Design review of the part built by this model. Coordinates are the model's own, in mm. A direction names the side the tool comes from. Coordinates: 2 decimals unless noted, no trailing zeros. Write each loop counter-clockwise with the first axis right and the second up, starting at its lowest first coordinate (ties: lowest second). Pieces come first, ordered by that corner, then holes. Notation, with made-up numbers: (-36, 79) - (-30, 79) arc R16 ccw to (-30, 89) - close; hole circle Ø1 at (22.25, -5.5). An arc over 180 degrees is marked (long way). One line per item, written item: value.
from build123d import *

# Parameters (mm, degrees)
SCHIZZO1_R                   = 1.5
ESTRUSIONE_ESTRUSIONE1_DEPTH = 4


with BuildPart() as part:
    # Schizzo1 → Estrusione-Estrusione1 (new body)
    with BuildSketch(Plane.XY):
        with BuildLine():
            Line((22.627416998, 28.387976608), (-22.627416998, 28.387976608))
            ThreePointArc((-22.627416998, 28.387976608), (-27.949480117, 24.831887722), (-26.700747761, 18.554086235))
            Line((-26.700747761, 18.554086235), (-4.073330763, -4.073330763))
            ThreePointArc((-4.073330763, -4.073330763), (0, -5.76055961), (4.073330763, -4.073330763))
            Line((4.073330763, -4.073330763), (26.700747761, 18.554086235))
            ThreePointArc((26.700747761, 18.554086235), (27.949480117, 24.831887722), (22.627416998, 28.387976608))
        make_face()
        Circle(SCHIZZO1_R, mode=Mode.SUBTRACT)
        with Locations((22.627416998, 22.627416998)):
            Circle(SCHIZZO1_R, mode=Mode.SUBTRACT)
        with Locations((-22.627416998, 22.627416998)):
            Circle(SCHIZZO1_R, mode=Mode.SUBTRACT)
        with BuildLine():
            Line((5.727922061, 17.627416998), (-5.727922061, 17.627416998))
            ThreePointArc((-5.727922061, 17.627416998), (-7.575681126, 16.392783863), (-7.142135624, 14.213203436))
            Line((-7.142135624, 14.213203436), (-1.414213562, 8.485281374))
            ThreePointArc((-1.414213562, 8.485281374), (0, 7.899494937), (1.414213562, 8.485281374))
            Line((1.414213562, 8.485281374), (7.142135624, 14.213203436))
            ThreePointArc((7.142135624, 14.213203436), (7.575681126, 16.392783863), (5.727922061, 17.627416998))
        make_face(mode=Mode.SUBTRACT)
    extrude(amount=ESTRUSIONE_ESTRUSIONE1_DEPTH)


solid = part.part
1. Consider section A-A, the plane z = 0.75. Write out the cut boundary in (x, y).
Answer block:
outline: (-26.7, 18.55) - (-4.07, -4.07) arc R5.76 ccw to (4.07, -4.07) - (26.7, 18.55) arc R5.76 ccw to (22.63, 28.39) - (-22.63, 28.39) arc R5.76 ccw to start; hole circle Ø3 at (-22.63, 22.63); hole (-7.14, 14.21) - (-1.41, 8.49) arc R2 ccw to (1.41, 8.49) - (7.14, 14.21) arc R2 ccw to (5.73, 17.63) - (-5.73, 17.63) arc R2 ccw to start; hole circle Ø3 at (0, 0); hole circle Ø3 at (22.63, 22.63)
2. For faces 4 (the face through (-15.545, 7.399, 1.972)), 5 (the face through (7.59, 16.36, 1.97)), list the 3-axis set-ups (+Z, -Z, +X, -X, +Y, -Y) from which the entire face can be reached by the end or side of a thin tool; tool diameter is ignored.
Answer block:
face 4: +Z, -Z, -X, -Y
face 5: +Z, -Z
3. Consider section D-D, the plane y = 16.5. Write out the cut boundary in (x, z).
Answer block:
outline: (-24.65, 0) - (-7.53, 0) - (-7.53, 4) - (-24.65, 4) - close; (7.53, 0) - (24.65, 0) - (24.65, 4) - (7.53, 4) - close
4. Wall thickness on line 1 along Y through (x, z) = (0, 2.1); line 2 along Y through (x, z) = (1, 1); line 3 along X through (y, z) = (22.5, 3.45): over which ranges is each line inside the solid? List them lowest first.
Answer block:
line 1: y = -5.76 to -1.5, 1.5 to 7.9, 17.63 to 28.39
line 2: y = -5.67 to -1.12, 1.12 to 8.17, 17.63 to 28.39
line 3: x = -28.39 to -24.12, -21.13 to 21.13, 24.12 to 28.39
5. Consider section B-B, the plane y = 0. Write out the cut boundary in (x, z).
Answer block:
outline: (-8.15, 0) - (-1.5, 0) - (-1.5, 4) - (-8.15, 4) - close; (1.5, 0) - (8.15, 0) - (8.15, 4) - (1.5, 4) - close
6. Mouldability with a two-part tool opening along Y and no side actions: class faces 1 (the face through (0, 19, 4)), 2 (the face through (0, 28.388, 2)), 3 (the face through (-1.5, 0.07, 1.97)) as released by +Y, released by -Y, zero draft, split by the parting line, or undercut.
Answer block:
face 1: zero draft
face 2: released by +Y
face 3: undercut
7. Consider section C-C, the plane x = 0. Write out the cut boundary in (y, z).
Answer block:
outline: (-5.76, 0) - (-1.5, 0) - (-1.5, 4) - (-5.76, 4) - close; (1.5, 0) - (7.9, 0) - (7.9, 4) - (1.5, 4) - close; (17.63, 0) - (28.39, 0) - (28.39, 4) - (17.63, 4) - close
8. Insertion check: pin 1 Ø1.2 at (x, z) = (-0.5, 2) entering from -Y; pin 2 Ø2 at (y, z) = (0, 2.5) entering from -X; pin 3 Ø2.5 at (x, y) = (22.63, 22.63) entering from +Z; pin 4 Ø1.5 at (y, z) = (11, 1) entering from -X. Each pin has a flat end and moves straight along its axis. Give the tip position at first contact, or say it passes through.
Answer block:
pin 1: stops at y = -5.76
pin 2: stops at x = -9.15
pin 3: passes through
pin 4: stops at x = -19.9
